For this review, take the finished solid that the model builds, in its own axes (mm). Give positions to 0.01 mm unless a question says otherwise; leave off trailing zeros. Order: outer loops, then holes, each group sorted by start corner. A loop starts at its lowest first (then second) coordinate and runs counter-clockwise, first axis right, second up. Notation, with made-up numbers: (-3.5, 2) -> (55.5, 2) arc R25 ccw to (55.5, 21) -> close; hole circle Ø3 at (-3, -17.5). An arc over 180 degrees is marked (long way). Return JSON: item names as keys, results as strings. Group by question number.
1) The part is to be moulded in two halves that separate along X. For faces 1 (the face through (64.952, -1, 99)), 2 (the face through (-64.952, 1, 99)), 3 (the face through (16.196, 5.1, 96.933)), 4 (the face through (5, 50, 0)), say which applies: released by +X, released by -X, zero draft, split by the parting line, or undercut.
2) To check wall thickness, follow line 1 along Y through (x, z) = (0, 105); line 2 along Y through (x, z) = (-30, 124); line 3 along X through (y, z) = (40.5, 187.5). State the ranges of each line that lie inside material, in increasing order.
3) Insertion check: P1, Ø3, axis at x = -17, z = 142.5, coming from the -Y side; P2, Ø1.5, axis at x = 29, y = 44, coming from the +Z side; P3, Ø8, axis at y = -57.5, z = 129.5, coming from the -X side. Each pin has a flat end and moves straight along its axis. Give the tip position at first contact, or say it passes through.
4) Add section A-A (z = 88). Give the boundary of the cut face in (x, y), then the cut area to 3 significant figures.
from build123d import *

# Parameters (mm, degrees)
F3_DEPTH = 206.616135


with BuildPart() as f1:
    # F0 (on Front) → F1 (revolve)
    with BuildSketch(Plane.XZ):
        with BuildLine():
            ThreePointArc((16.980399, 84.057986), (46.830312, 47.269247), (50, 0))
            Line((50, 0), (75, 0))
            Line((75, 0), (75, 200))
            Line((75, 200), (50.020899, 198.977988))
            ThreePointArc((50.020899, 198.977988), (48.457809, 149.011176), (16.980399, 110.174363))
            Line((16.980399, 110.174363), (16.980399, 84.057986))
        make_face()
    revolve(axis=Axis((0, 0, 42.679031), (0, 0, 1)))

    # F2 (on Top) → F3 (intersect)
    with BuildSketch(Plane.XY):
        Polygon((-64.951905, 37.5), (-64.951905, -37.5), (0, -75), (64.951905, -37.5), (64.951905, 37.5), (0, 75), align=None)
    extrude(amount=F3_DEPTH, mode=Mode.INTERSECT)


solid = f1.part
Evaluation:
{
 "1": {"face 1": "released by +X", "face 2": "released by -X", "face 3": "undercut", "face 4": "zero draft"},
 "2": {"line 1": "-75 to -16.98, 16.98 to 75", "line 2": "-57.68 to -14.52, 14.52 to 57.68", "line 3": "-59.76 to -33.52, 33.52 to 59.76"},
 "3": {"P1": "y = -66.05", "P2": "z = 199.12", "P3": "x = -37.24"},
 "4": {"outline": "(-64.95, -37.5) -> (0, -75) -> (64.95, -37.5) -> (64.95, 37.5) -> (0, 75) -> (-64.95, 37.5) -> close; hole circle Ø33.96 at (0, 0)", "area": "13,700 mm^2"}
}
